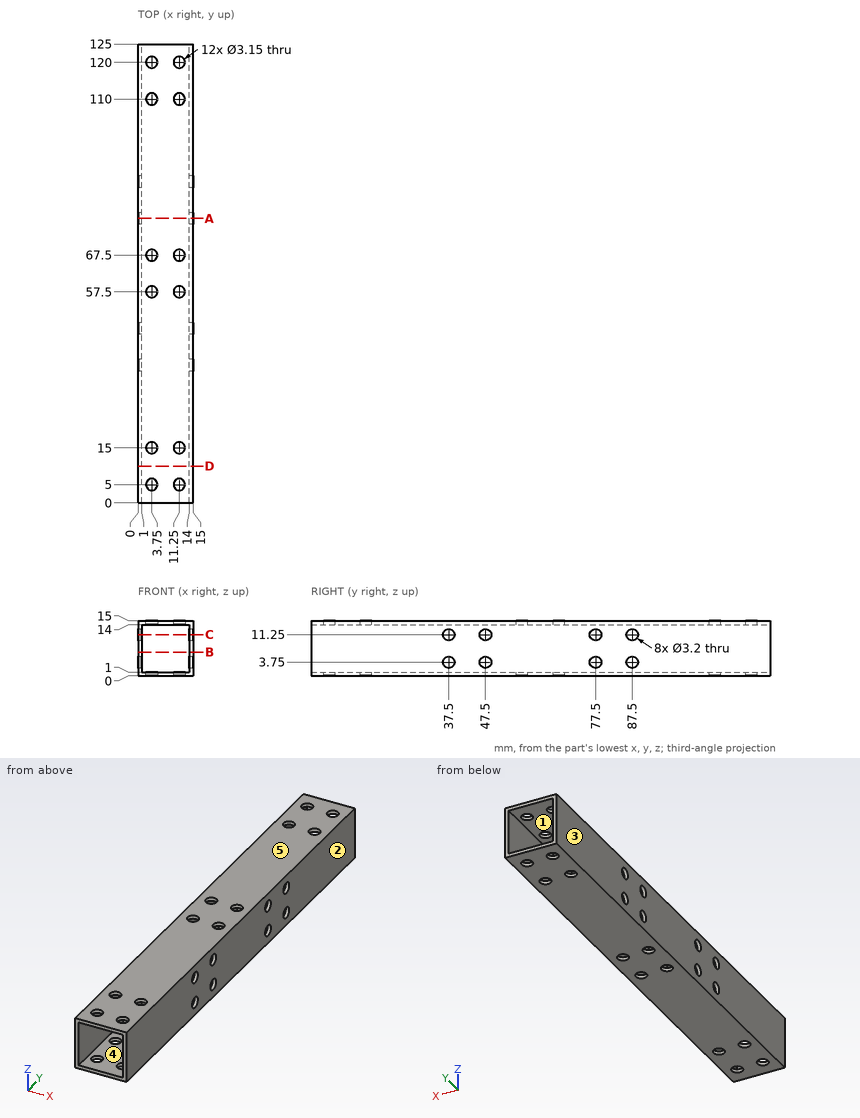
Geometry: see drawing. Coordinates: mm, zero at the bounding-box minimum. A direction names the side the tool comes from. Round coordinates to 2 decimals unless told otherwise and drop trailing zeros. Order: outer loops, then holes, each group sorted by start corner. A loop starts at its lowest first (then second) coordinate and runs counter-clockwise, first axis right, second up. Notation, with made-up numbers: (36.25, 80.25) - (57.25, 80.25) arc R24 cw to (57.25, 101.25) - close; hole circle Ø4 at (11.25, 34.25). An arc over 180 degrees is marked (long way). Use a Markdown table: item, result. Add a question column.
1. Section query D-D (y = 10). Return the cut outline in (x, z), then the cut area to 3 significant figures.
2. Section query C-C (z = 11.25). Give the number of separate pieces and of enclosed holes in the cut face, then the cut area to 3 significant figures.
3. First-contact query: pin 1 (2.5 mm diameter, centred on y = 47.5, z = 3.75, fed in from +X) (3 decimals). Flat tip, straight axial feed; report the tip coordinate or a pass-through.
4. Line query: probe 1 along X at (y, z) = (120, 14.3) (3 decimals); probe 2 along Y at (x, z) = (14.7, 3.75); probe 3 along Z at (x, y) = (8.5, 87.5). Output: solid intervals per line, ascending.
5. Section query A-A (y = 77.5). Return the cut outline in (x, z), then the cut area to 3 significant figures.
6. Set-up query: the marked faces 4 and 5. Return all of +Z, -Z, +X, -X, +Y, -Y with unobstructed straight access to the full face (end or side cutting, diameter ignored); none if empty.
7. Section query B-B (z = 6.5). Return the cut outline in (x, y), then the cut area to 3 significant figures.
8. Mould query, pull axis X, two halves, no side actions, for the marked faces 1, 2 and 3. Classes: +X half, -X half, draft (parallel to the pull), parting line (faces both ways), or undercut.
Derived:
| question | item | result |
|---|---|---|
| 1 | outline | (0, 0) - (15, 0) - (15, 15) - (0, 15) - close; hole (1, 1) - (14, 1) - (14, 14) - (1, 14) - close |
| 1 | area | 56.0 mm2 |
| 2 | separate pieces | 10 |
| 2 | enclosed holes | 0 |
| 2 | area | 224 mm2 |
| 3 | pin 1 | through |
| 4 | probe 1 | 0 to 2.175, 5.325 to 9.675, 12.825 to 15 |
| 4 | probe 2 | 0 to 35.9, 39.1 to 45.9, 49.1 to 75.9, 79.1 to 85.9, 89.1 to 125 |
| 4 | probe 3 | 0 to 1, 14 to 15 |
| 5 | outline | (0, 0) - (15, 0) - (15, 2.15) - (14, 2.15) - (14, 1) - (1, 1) - (1, 2.15) - (0, 2.15) - close; (0, 5.35) - (1, 5.35) - (1, 9.65) - (0, 9.65) - close; (0, 12.85) - (1, 12.85) - (1, 14) - (14, 14) - (14, 12.85) - (15, 12.85) - (15, 15) - (0, 15) - close; (14, 5.35) - (15, 5.35) - (15, 9.65) - (14, 9.65) - close |
| 5 | area | 43.2 mm2 |
| 6 | face 4 | +Y, -Y |
| 6 | face 5 | +Z, +X, -X, +Y, -Y |
| 7 | outline | (0, 0) - (1, 0) - (1, 125) - (0, 125) - close; (14, 0) - (15, 0) - (15, 125) - (14, 125) - close |
| 7 | area | 250 mm2 |
| 8 | face 1 | undercut |
| 8 | face 2 | +X half |
| 8 | face 3 | -X half |
